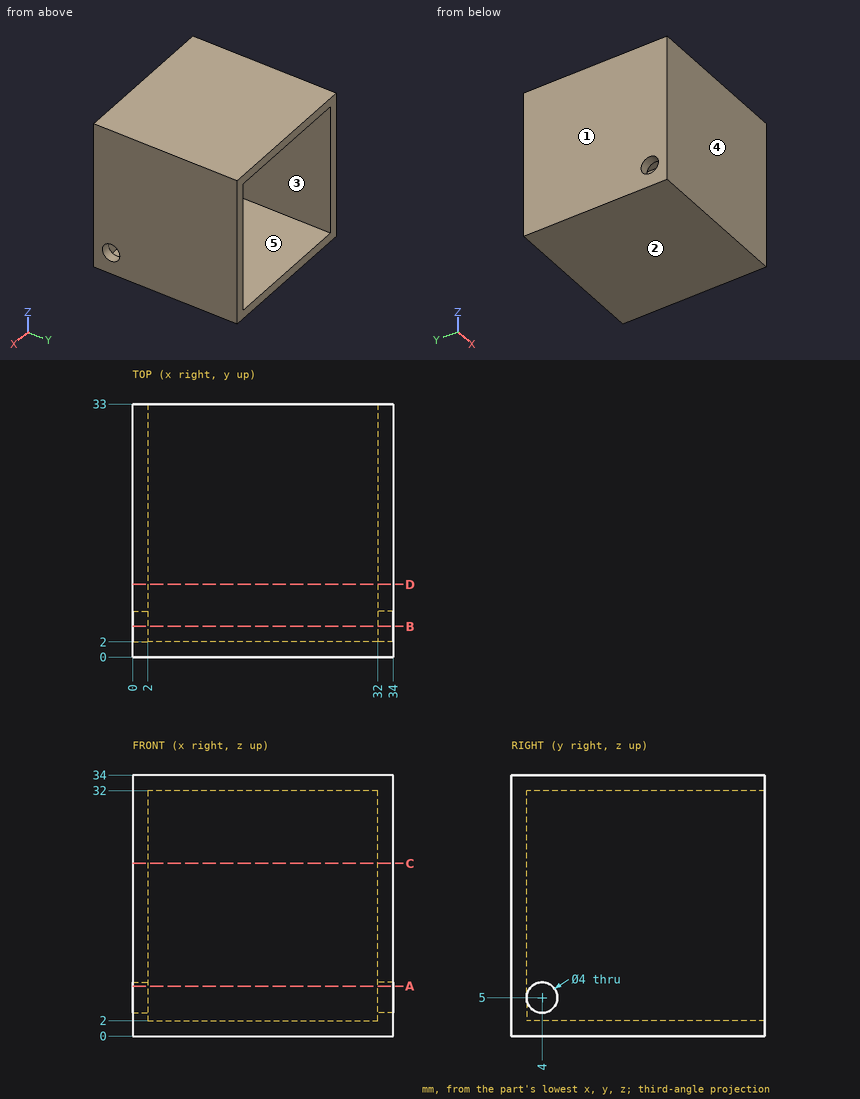
Design review of the part shown in the three views and the two pictorial views. Dimensions are in mm from the part's minimum x, y and z. A direction names the side the tool comes from. Round coordinates to 2 decimals unless told otherwise and drop trailing zeros. Loops run counter-clockwise (first coordinate to the right, second up) from the corner with the lowest first, then second, coordinate; pieces in that order, holes last. Notation, with made-up numbers: (86.5, 3.25) -> (98.5, 3.25) arc R18 ccw to (98.5, 35.25) -> close; hole circle Ø9 at (-5, 17). An arc over 180 degrees is marked (long way). Answer as a JSON object with one key per item and string values. Group by question number.
1) For pin 1 Ø10 at (x, z) = (14.5, 22.5) entering from +Y, flat-tipped, find the tip position at first contact; note if it passes through.
2) For line 1 (Y direction, x = 33, z = 5); line 2 (Z direction, x = 0.5, y = 4); line 3 (X direction, y = 21, z = 31), list the stretches that pass through material, from the lowest coordinate up. Write a range as [from, to].
3) We need section B-B on y = 4. Write out the cut boundary in (x, z), then the cut area to 3 significant figures.
4) We need section A-A on z = 6.5. Write out the cut boundary in (x, y), then the cut area to 3 significant figures.
5) For the marked faces 4 and 5, list the 3-axis set-ups (+Z, -Z, +X, -X, +Y, -Y) from which the entire face can be reached by the end or side of a thin tool; tool diameter is ignored.
6) Mouldability with a two-part tool opening along X and no side actions: class the marked faces 1, 2 and 3 as released by +X, released by -X, zero draft, split by the parting line, or undercut.
7) We need section D-D on y = 9.5. Write out the cut boundary in (x, z), then the cut area to 3 significant figures.
8) We need section C-C on z = 22.5. Write out the cut boundary in (x, y), then the cut area to 3 significant figures.
Result set:
{
 "1": {"pin 1": "y = 2"},
 "2": {"line 1": "[0, 2], [6, 33]", "line 2": "[0, 3], [7, 34]", "line 3": "[0, 2], [32, 34]"},
 "3": {"outline": "(0, 0) -> (34, 0) -> (34, 3) -> (32, 3) -> (32, 2) -> (2, 2) -> (2, 3) -> (0, 3) -> close; (0, 7) -> (2, 7) -> (2, 32) -> (32, 32) -> (32, 7) -> (34, 7) -> (34, 34) -> (0, 34) -> close", "area": "240 mm²"},
 "4": {"outline": "(0, 0) -> (34, 0) -> (34, 2.68) -> (32, 2.68) -> (32, 2) -> (2, 2) -> (2, 2.68) -> (0, 2.68) -> close; (0, 5.32) -> (2, 5.32) -> (2, 33) -> (0, 33) -> close; (32, 5.32) -> (34, 5.32) -> (34, 33) -> (32, 33) -> close", "area": "181 mm²"},
 "5": {"face 4": "+Z, -Z, +X, -X, -Y", "face 5": "+Y"},
 "6": {"face 1": "released by -X", "face 2": "zero draft", "face 3": "undercut"},
 "7": {"outline": "(0, 0) -> (34, 0) -> (34, 34) -> (0, 34) -> close; hole (2, 2) -> (32, 2) -> (32, 32) -> (2, 32) -> close", "area": "256 mm²"},
 "8": {"outline": "(0, 0) -> (34, 0) -> (34, 33) -> (32, 33) -> (32, 2) -> (2, 2) -> (2, 33) -> (0, 33) -> close", "area": "192 mm²"}
}
